Part model, mm, in its own coordinate system. A direction names the side the tool comes from. Give positions to 0.01 mm unless a question says otherwise; leave off trailing zeros. Order: outer loops, then holes, each group sorted by start corner. A loop starts at its lowest first (then second) coordinate and runs counter-clockwise, first axis right, second up. Notation, with made-up numbers: (20.5, 69.5) - (32.5, 69.5) arc R11 cw to (32.5, 89.5) - close; hole circle Ø8 at (33, -9). An arc over 180 degrees is marked (long way). One line per item, written item: value.
```python
from build123d import *

# Parameters (mm, degrees)
EXTRUDE_1_DEPTH = 3
SKETCH_2_R      = 1.75
EXTRUDE_2_DEPTH = 4.5


with BuildPart() as part:
    # 草图1 → 凸台-拉伸1 (new body)
    with BuildSketch(Plane(origin=(0, 0, 0), x_dir=(1, 0, 0), z_dir=(0, 1, 0))):
        with BuildLine():
            Line((-2.8, -3), (2.8, -3))
            ThreePointArc((2.8, -3), (2.941421356, -2.941421356), (3, -2.8))
            Line((3, -2.8), (3, 2.8))
            ThreePointArc((3, 2.8), (2.941421356, 2.941421356), (2.8, 3))
            Line((2.8, 3), (-2.8, 3))
            ThreePointArc((-2.8, 3), (-2.941421356, 2.941421356), (-3, 2.8))
            Line((-3, 2.8), (-3, -2.8))
            ThreePointArc((-3, -2.8), (-2.941421356, -2.941421356), (-2.8, -3))
        make_face()
    extrude(amount=EXTRUDE_1_DEPTH)

    # 草图2 → 凸台-拉伸2 (add)
    with BuildSketch(Plane(origin=(0, 3, 0), x_dir=(1, 0, 0), z_dir=(0, 1, 0))):
        Circle(SKETCH_2_R)
    extrude(amount=EXTRUDE_2_DEPTH)


solid = part.part
```
1) Which spindle directions (+Z, -Z, +X, -X, +Y, -Y) get a long thin tool onto all of the face, cutting with end or side? Do faces 1 (the flat face through (0, 0, 0)), 2 (the cylindrical face through (1.617, 5.219, 0.67)). Say none if no direction does.
Outcome:
face 1: +Z, -Z, +X, -X, -Y
face 2: +Y
2) Cut at D-D, the plane x = -2.4. Give the cut face in (y, z).
Outcome:
outline: (0, -3) - (3, -3) - (3, 3) - (0, 3) - close
3) Cut at C-C, the plane y = 3.25. Give the cut face in (x, z), then the cut area to 3 significant figures.
Outcome:
outline: circle Ø3.5 at (0, 0)
area: 9.62 mm^2
4) Pin check, flat tips, straight feed: pin 1 (3 mm diameter, centred on x = 1, z = 0.5, fed in from -Y); pin 2 (1.5 mm diameter, centred on y = 5, z = -2, fed in from +X). Stop position of each tip, or through.
Outcome:
pin 1: stops at y = 0
pin 2: stops at x = 1.22
5) Cut at A-A, the plane x = 1.4. Give the cut face in (y, z), then the cut area to 4 significant figures.
Outcome:
outline: (0, -3) - (3, -3) - (3, -1.05) - (7.5, -1.05) - (7.5, 1.05) - (3, 1.05) - (3, 3) - (0, 3) - close
area: 27.45 mm^2
6) Cut at B-B, the plane z = 0. Give the cut face in (x, y), then the cut area to 4 significant figures.
Outcome:
outline: (-3, 0) - (3, 0) - (3, 3) - (1.75, 3) - (1.75, 7.5) - (-1.75, 7.5) - (-1.75, 3) - (-3, 3) - close
area: 33.75 mm^2
7) Drill centre lines: line 1 along Y through (x, z) = (-2.2, -2.25); line 2 along Z through (x, y) = (0.1, 6.25). Where is each one in solid material? Low to high. Write a range as from..to.
Outcome:
line 1: y = 0..3
line 2: z = -1.75..1.75
